Print and shaded views of the part. All mm, measured from the part's lowest x, y and z. Give positions to 0.01 mm unless a question says otherwise; leave off trailing zeros. Loops run counter-clockwise (first coordinate to the right, second up) from the corner with the lowest first, then second, coordinate; pieces in that order, holes last. Notation, with made-up numbers: M -34,25 L -24,25 A22 cw -24,33 Z; hole C 8,48.25 d4. An arc over 180 degrees is marked long. Answer in a Markdown table with one row per item.
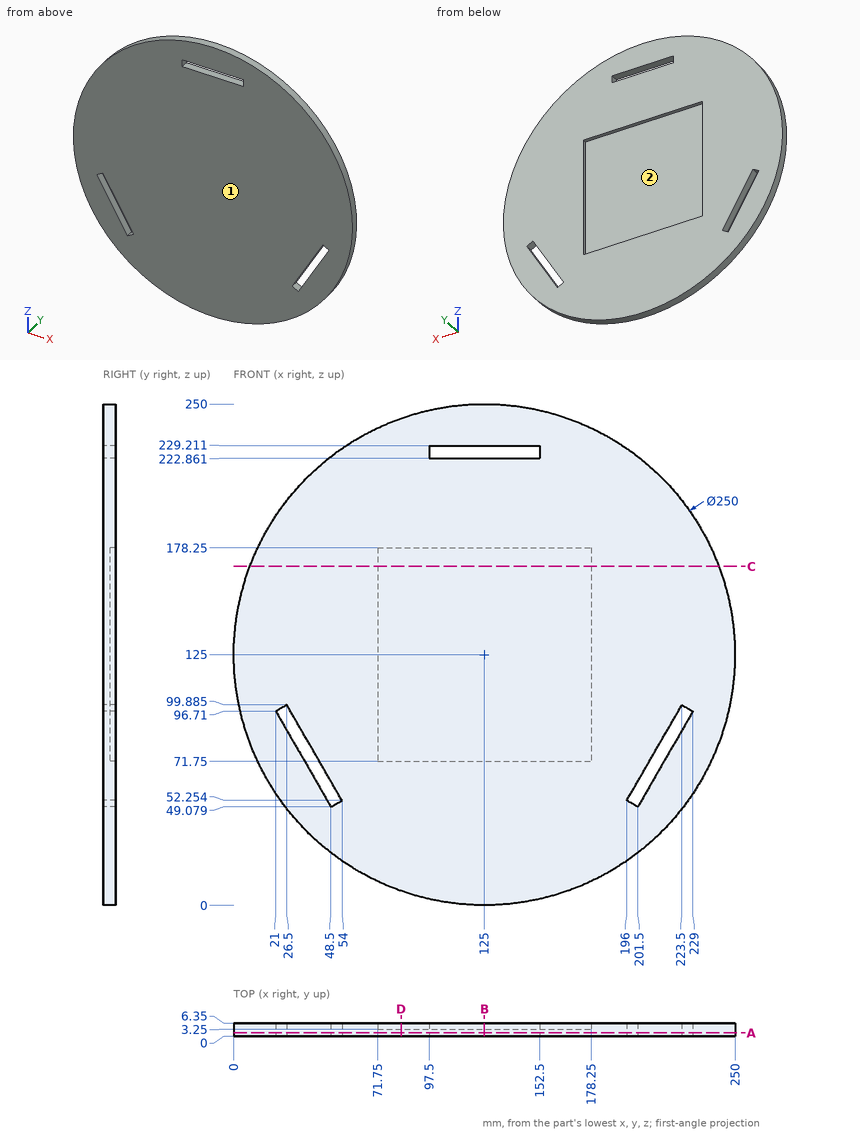
(1) Saw through at B-B, the plane x = 125. Give the cut face in (y, z), and give its area (3 significant figures).
Established:
| item | result |
|---|---|
| outline | M 0,0 L 6.35,0 L 6.35,71.75 L 3.25,71.75 L 3.25,178.25 L 6.35,178.25 L 6.35,222.86 L 0,222.86 Z; M 0,229.21 L 6.35,229.21 L 6.35,250 L 0,250 Z |
| area | 1,220 mm2 |
(2) Saw through at D-D, the plane x = 83.5. Give the cut face in (y, z), and give its area (3 significant figures).
Established:
| item | result |
|---|---|
| outline | M 0,7.09 L 6.35,7.09 L 6.35,71.75 L 3.25,71.75 L 3.25,178.25 L 6.35,178.25 L 6.35,242.91 L 0,242.91 Z |
| area | 1,170 mm2 |
(3) Saw through at A-A, the plane y = 1.5. Give the cut face in (x, z) (1 decimal), and give its area (3 significant figures).
Established:
| item | result |
|---|---|
| outline | C 125,125 d250; hole M 21,96.7 L 48.5,49.1 L 54,52.3 L 26.5,99.9 Z; hole M 97.5,222.9 L 152.5,222.9 L 152.5,229.2 L 97.5,229.2 Z; hole M 196,52.3 L 201.5,49.1 L 229,96.7 L 223.5,99.9 Z |
| area | 48,000 mm2 |
(4) Flat gauge pins, fed straight in: P1, Ø3.5, axis at x = 116.5, y = 5.5, coming from the +Z side; P2, Ø3, axis at y = 2.5, z = 226.5, coming from the +X side; P3, Ø1.6, axis at y = 4, z = 150, coming from the -X side (1 decimal); P4, Ø4, axis at x = 213, z = 218.5, coming from the +Y side. Where does each tip first touch, or does it go through?
Established:
| item | result |
|---|---|
| P1 | stops at z = 249.82 |
| P2 | stops at x = 200 |
| P3 | stops at x = 2.4 |
| P4 | passes through |
(5) Saw through at C-C, the plane z = 169. Give the cut face in (x, y), and give its area (3 significant figures).
Established:
| item | result |
|---|---|
| outline | M 8,0 L 242,0 L 242,6.35 L 178.25,6.35 L 178.25,3.25 L 71.75,3.25 L 71.75,6.35 L 8,6.35 Z |
| area | 1,160 mm2 |
(6) Mould opens along Z. For the marked faces 1 and 2 say: pulls with the +Z half, pulls with the -Z half, needs draft (parallel to the pull), parting line crosses it, or undercut.
Established:
| item | result |
|---|---|
| face 1 | needs draft |
| face 2 | undercut |
(7) Wall check: L1, parallel to X at y = 5.75, z = 76.5; L2, parallel to Z at x = 105.5, y = 6; L3, parallel to X at y = 1.75, z = 49.5 (1 decimal). Give the ranges that are in metal, low to high.
Established:
| item | result |
|---|---|
| L1 | x = 9.79 to 32.67, 40 to 71.75, 178.25 to 210, 217.33 to 240.21 |
| L2 | z = 1.53 to 71.75, 178.25 to 222.86, 229.21 to 248.47 |
| L3 | x = 25.4 to 48.3, 49.2 to 200.8, 201.7 to 224.6 |
